The model under review builds one solid part; all positions refer to its coordinate system, in mm. A direction names the side the tool comes from. Give positions to 0.01 mm unless a question says otherwise; leave off trailing zeros. Loops run counter-clockwise (first coordinate to the right, second up) from the corner with the lowest first, then second, coordinate; pieces in that order, holes last. Notation, with made-up numbers: (-19, 59) - (28, 59) arc R14 cw to (28, 67) - close; hole circle Ø4 at (37, -0.75). An arc over 180 degrees is marked (long way). Answer as a JSON object with one key per item and string values.
from build123d import *

# Parameters (mm, degrees)
SALIENTE_EXTRUIR1_DEPTH = 10
CROQUIS1_10_R           = 3.9
CORTAR_EXTRUIR1_DEPTH   = 6
CROQUIS1_11_R           = 1.55
CORTAR_EXTRUIR3_DEPTH   = 283.658804922


with BuildPart() as part:
    # Croquis1 → Saliente-Extruir1 (new body)
    with BuildSketch(Plane(origin=(0, 0, 0), x_dir=(1, 0, 0), z_dir=(0, 1, 0))):
        Polygon((0, 0), (20, 0), (20, -12), (48, -12), (48, 0), (68, 0), (68, -12), (96, -12), (96, 0), (116, 0), (116, -12), (144, -12), (144, 0), (164, 0), (164, 230), (0, 230), align=None)
    extrude(amount=SALIENTE_EXTRUIR1_DEPTH)

    # Croquis1_10 → Cortar-Extruir1 (cut)
    with BuildSketch(Plane(origin=(0, 0, 0), x_dir=(1, 0, 0), z_dir=(0, 1, 0))):
        with Locations(Location((62, 190, 0), (0, 0, 270))):
            Circle(CROQUIS1_10_R)
        with Locations(Location((102, 190, 0), (0, 0, 270))):
            Circle(CROQUIS1_10_R)
    extrude(amount=CORTAR_EXTRUIR1_DEPTH, mode=Mode.SUBTRACT)

    # Croquis1_11 → Cortar-Extruir3 (cut, through all)
    with BuildSketch(Plane(origin=(0, 0, 0), x_dir=(1, 0, 0), z_dir=(0, 1, 0))):
        with Locations(Location((107, 155, 0), (0, 0, 270))):
            Circle(CROQUIS1_11_R)
    extrude(amount=CORTAR_EXTRUIR3_DEPTH, mode=Mode.SUBTRACT)


solid = part.part
Q1. The part is to be moulded in two halves that separate along Z. For faces 1 (the face through (82, 5, 12)), 2 (the face through (62, 6, -190)), 3 (the face through (164, 5, -113)), say which applies: +Z half, -Z half, draft (parallel to the pull), parting line (faces both ways), or undercut.
Results:
{"face 1": "+Z half", "face 2": "undercut", "face 3": "draft"}
Q2. Consider section A-A, the plane z = -190. State the section outline as (x, y) points, plus the area to 3 significant figures.
Results:
{"outline": "(0, 0) - (58.1, 0) - (58.1, 6) - (65.9, 6) - (65.9, 0) - (98.1, 0) - (98.1, 6) - (105.9, 6) - (105.9, 0) - (164, 0) - (164, 10) - (0, 10) - close", "area": "1,550 mm^2"}
Q3. For faces 4 (the face through (106, 5, 0)), 5 (the face through (34, 5, 12)), 6 (the face through (20, 5, 6)), 7 (the face through (154, 5, 0)), 8 (the face through (99.627, 2.958, -193.095)), list the 3-axis set-ups (+Z, -Z, +X, -X, +Y, -Y) from which the entire face can be reached by the end or side of a thin tool; tool diameter is ignored.
Results:
{"face 4": "+Z, +Y, -Y", "face 5": "+Z, +X, -X, +Y, -Y", "face 6": "+Z, -X, +Y, -Y", "face 7": "+Z, +X, +Y, -Y", "face 8": "-Y"}
Q4. Consider section B-B, the plane x = 102. State the section outline as (y, z) points, plus the area to 3 significant figures.
Results:
{"outline": "(0, -230) - (10, -230) - (10, 0) - (0, 0) - (0, -186.1) - (6, -186.1) - (6, -193.9) - (0, -193.9) - close", "area": "2,250 mm^2"}
Q5. To check wall thickness, follow probe 1 along X at (y, z) = (2.8, -190); probe 2 along X at (y, z) = (7.25, -155); probe 3 along Z at (x, y) = (107, 2.5). State the ranges of each line that lie inside material, in increasing order. Write a range as [from, to].
Results:
{"probe 1": "x = [0, 58.1], [65.9, 98.1], [105.9, 164]", "probe 2": "x = [0, 105.45], [108.55, 164]", "probe 3": "z = [-230, -156.55], [-153.45, 0]"}
Q6. Clearance check with flat-ended pins moving along their axes: pin 1 Ø4 at (x, z) = (63.5, -189.5) entering from -Y; pin 2 Ø5 at (x, y) = (55, 7) entering from +Z; pin 3 Ø1.5 at (y, z) = (3, -148.5) entering from -X; pin 4 Ø5 at (y, z) = (4.5, 7.5) entering from +X. State where each tip first meets the part, or that it passes through.
Results:
{"pin 1": "stops at y = 6", "pin 2": "stops at z = 0", "pin 3": "stops at x = 0", "pin 4": "stops at x = 144"}
